For this review, take the finished solid that the model builds, in its own axes (mm). Face numbers are marked on the shaded views. A direction names the side the tool comes from. Give positions to 0.01 mm unless a question says otherwise; leave off trailing zeros. Order: outer loops, then holes, each group sorted by start corner. A loop starts at its lowest first (then second) coordinate and runs counter-clockwise, first axis right, second up. Notation, with made-up numbers: (5, 67.25) - (19, 67.25) arc R8 ccw to (19, 74.25) - close; hole circle Ø10 at (-19, -1). An arc over 180 degrees is marked (long way). Answer as a JSON object with one key per item and string values. Group by question number.
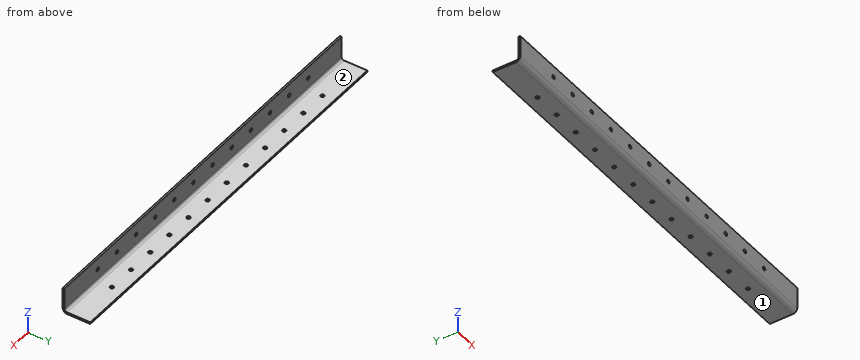
from build123d import *

# Parameters (mm, degrees)
SKETCH1_W                    = 2200
SKETCH1_H                    = 150
BASE_FLANGE1_DEPTH           = 10
EDGE_FLANGE1_STRIP_W         = 68
EDGE_FLANGE1_STRIP_H         = 10
EDGE_FLANGE1_STRIP_CUT_DEPTH = 2200
EDGE_FLANGE1_DEPTH           = 2200
SKETCH12_R                   = 10
CUT_EXTRUDE1_DEPTH           = 10
SKETCH13_R                   = 10
CUT_EXTRUDE2_DEPTH           = 10
LPATTERN1_COUNT              = 12
LPATTERN1_PITCH              = 152


# Sheet-metal steps are written as plain solids
with BuildPart() as part:
    # Sketch1 → Base-Flange1 (new body)
    with BuildSketch(Plane.XY):
        Rectangle(SKETCH1_W, SKETCH1_H)
    extrude(amount=-BASE_FLANGE1_DEPTH)

    # Edge-Flange1 strip (across the edge) → Edge-Flange1 strip cut (cut)
    with BuildSketch(Plane(origin=(-1100, -75, 0), x_dir=(0, 1, 0), z_dir=(1, 0, 0))):
        with Locations((-10, -5)):
            Rectangle(EDGE_FLANGE1_STRIP_W, EDGE_FLANGE1_STRIP_H)
    extrude(amount=EDGE_FLANGE1_STRIP_CUT_DEPTH, mode=Mode.SUBTRACT)

    # Edge-Flange1 section (across the edge) → Edge-Flange1 (add)
    with BuildSketch(Plane(origin=(-1100, -75, 0), x_dir=(0, 1, 0), z_dir=(1, 0, 0))):
        with BuildLine():
            Line((0, 14), (0, 130))
            Line((0, 130), (10, 130))
            Line((10, 130), (10, 14))
            ThreePointArc((10, 14), (14.100505063, 4.100505063), (24, 0))
            Line((24, 0), (24, -10))
            ThreePointArc((24, -10), (7.029437252, -2.970562748), (0, 14))
        make_face()
    extrude(amount=EDGE_FLANGE1_DEPTH)

    # Sketch12 → Cut-Extrude1 (cut)
    with BuildSketch(Plane(origin=(0, -75, 0), x_dir=(-1, 0, 0), z_dir=(0, -1, 0))):
        with Locations(Location((836, -67, 0), (0, 0, 90))):
            Circle(SKETCH12_R)
    cut_extrude1 = extrude(amount=-CUT_EXTRUDE1_DEPTH, mode=Mode.SUBTRACT)

    # Sketch13 → Cut-Extrude2 (cut)
    with BuildSketch(Plane(origin=(0, 0, -10), x_dir=(-1, 0, 0), z_dir=(0, 0, -1))):
        with Locations((836, 12)):
            Circle(SKETCH13_R)
    cut_extrude2 = extrude(amount=-CUT_EXTRUDE2_DEPTH, mode=Mode.SUBTRACT)

    # LPattern1: Cut-Extrude1, Cut-Extrude2 ×12
    with Locations(*[(i * LPATTERN1_PITCH, 0, 0) for i in range(1, LPATTERN1_COUNT)]):
        add(cut_extrude1, mode=Mode.SUBTRACT)
        add(cut_extrude2, mode=Mode.SUBTRACT)


solid = part.part
1) Consider section A-A (x = -7.5). Give the boundary of the cut face in (y, z), plus the area to 3 significant figures.
2) Consider section B-B (y = 41). Give the boundary of the cut face in (x, z).
3) For pin 1 (6 mm diameter, centred on x = -73.5, y = 38.5, fed in from +Z); pin 2 (12 mm diameter, centred on x = -380, y = 12, fed in from -Z); pin 3 (8 mm diameter, centred on x = -409, z = 84.5, fed in from +Y); pin 4 (6 mm diameter, centred on x = -552.5, z = 8.5, fed in from -Y), all flat-tipped, find the tip position at first contact; note any pin that passes through.
4) For line 1 (Y direction, x = 934, z = 13); line 2 (Z direction, x = -83, y = 55); line 3 (Z direction, x = -228, y = -69.25), list the stretches that pass through material, from the lowest coordinate up.
5) For the marked faces 1 and 2, list the 3-axis set-ups (+Z, -Z, +X, -X, +Y, -Y) from which the entire face can be reached by the end or side of a thin tool; tool diameter is ignored.
Result set:
{
 "1": {"outline": "(-75, 14) arc R24 ccw to (-51, -10) - (75, -10) - (75, 0) - (-51, 0) arc R14 cw to (-65, 14) - (-65, 130) - (-75, 130) - close", "area": "2,720 mm2"},
 "2": {"outline": "(-1100, -10) - (1100, -10) - (1100, 0) - (-1100, 0) - close"},
 "3": {"pin 1": "stops at z = 0", "pin 2": "passes through", "pin 3": "stops at y = -65", "pin 4": "stops at y = -74.87"},
 "4": {"line 1": "y = -74.98 to -64.96", "line 2": "z = -10 to 0", "line 3": "z = -1.59 to 57, 77 to 130"},
 "5": {"face 1": "-Z, +X, -X, +Y, -Y", "face 2": "+Z, +X, -X, +Y"}
}
